Part model, mm, in its own coordinate system. Face numbers are marked on the shaded views. A direction names the side the tool comes from. Coordinates: 2 decimals unless noted, no trailing zeros. Order: outer loops, then holes, each group sorted by start corner. A loop starts at its lowest first (then second) coordinate and runs counter-clockwise, first axis right, second up.
1) Pin check, flat tip, straight feed: pin 1 Ø15 at (x, y) = (73, 36) entering from +Z. Stop position of the tip, or through.
2) Wall check: L1, parallel to Y at x = -72.5, z = 23; L2, parallel to X at y = 70.5, z = 8; L3, parallel to Z at x = 71, y = 161.5. Give the ranges that are in metal, low to high.
3) Cut at C-C (y = 167). List the corners of the cut face in (x, z).
4) Cut at D-D (x = 101.5). List the corners of the cut face in (y, z), and give its area (3 significant figures).
5) Tool access for the marked faces 4, 5 and 6: list every direction of +Z, -Z, +X, -X, +Y, -Y with a clear straight run to the whole face (end or side of a thin tool).
6) Mould opens along Y. For the marked faces 1, 2 and 3 say: +Y half, -Y half, draft (parallel to the pull), parting line (faces both ways), or undercut.
7) Cut at A-A (z = 29). List the corners of the cut face in (x, y), and give its area (3 significant figures).
8) Cut at B-B (x = 56.5). List the corners of the cut face in (y, z), and give its area (3 significant figures).
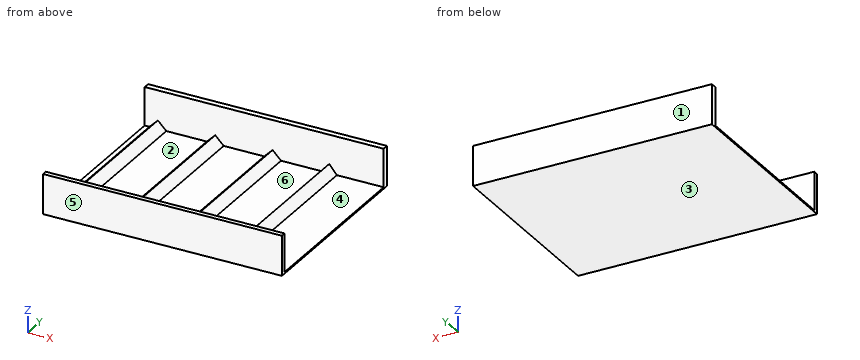
```python
from build123d import *

# Parameters (mm, degrees)
F0_W     = 300
F0_H     = 240
F1_DEPTH = 50
F2_W     = 300
F2_H     = 226.181105
F3_DEPTH = 48
F5_DEPTH = 228.9


with BuildPart() as f1:
    # F0 (on Top) → F1 (new body)
    with BuildSketch(Plane.XY):
        with Locations((14.745144, 69.408495)):
            Rectangle(F0_W, F0_H)
    extrude(amount=F1_DEPTH)

    # F2 (on face) → F3 (cut)
    with BuildSketch(Plane.XY.offset(50)):
        with Locations((14.745144, 68.680338)):
            Rectangle(F2_W, F2_H)
    extrude(amount=-F3_DEPTH, mode=Mode.SUBTRACT)

    # F4 (on face) → F5 (join)
    with BuildSketch(Plane.XZ.offset(-181.770891)):
        Polygon((-118.691458, 12.606602), (-129.298059, 2), (-108.084856, 2), align=None)
        Polygon((14.745144, 2), (35.958348, 2), (25.351746, 12.606602), align=None)
        Polygon((86.758348, 2), (106.004746, 2), (96.381547, 13.506261), align=None)
        Polygon((-57.284856, 2), (-36.054856, 2), (-46.669856, 12.598197), align=None)
    extrude(amount=F5_DEPTH)


solid = f1.part
```
Geometry check:
1. pin 1: stops at z = 2
2. L1: y = -50.59 to -44.41, 181.77 to 189.41
2. L2: x = -123.3 to -114.08, -51.28 to -42.06, 20.75 to 29.96, 91.78 to 100.99
2. L3: z = 0 to 2
3. outline: (-135.25, 0) - (164.75, 0) - (164.75, 2) - (106, 2) - (96.38, 13.51) - (86.76, 2) - (35.96, 2) - (25.35, 12.61) - (14.75, 2) - (-36.05, 2) - (-46.67, 12.6) - (-57.28, 2) - (-108.08, 2) - (-118.69, 12.61) - (-129.3, 2) - (-135.25, 2) - close
4. outline: (-50.59, 0) - (189.41, 0) - (189.41, 50) - (181.77, 50) - (181.77, 7.39) - (-44.41, 7.39) - (-44.41, 50) - (-50.59, 50) - close
4. area: 2,360 mm2
5. face 4: +Z, +X
5. face 5: +Z, -Z, +X, -X, -Y
5. face 6: +Z
6. face 1: +Y half
6. face 2: undercut
6. face 3: draft
7. outline: (-135.25, -50.59) - (164.75, -50.59) - (164.75, -44.41) - (-135.25, -44.41) - close; (-135.25, 181.77) - (164.75, 181.77) - (164.75, 189.41) - (-135.25, 189.41) - close
7. area: 4,150 mm2
8. outline: (-50.59, 0) - (189.41, 0) - (189.41, 50) - (181.77, 50) - (181.77, 2) - (-44.41, 2) - (-44.41, 50) - (-50.59, 50) - close
8. area: 1,140 mm2
